Here's how the part is built. I have some questions about the finished solid (model axes, mm). Face numbers are marked on the shaded views. A direction names the side the tool comes from. Round coordinates to 2 decimals unless told otherwise and drop trailing zeros. Loops run counter-clockwise (first coordinate to the right, second up) from the corner with the lowest first, then second, coordinate; pieces in that order, holes last. Notation, with made-up numbers: M 24,72 L 58,72 A12 ccw 58,82 Z; hole C -13,-15.5 d11. An arc over 180 degrees is marked long. Write item = value, one per line. Start each with the question number.
from build123d import *

# Parameters (mm, degrees)
F0_W        = 60
F0_H        = 70
F0_W_2      = 50
F0_H_2      = 60
F1_DEPTH    = 25
F1_FACE_W   = 60
F1_FACE_H   = 70
F1_FACE_W_2 = 50
F1_FACE_H_2 = 60
F2_DEPTH    = 60
F3_R        = 5
F4_R        = 3.5
F5_DEPTH    = 70


with BuildPart() as f1:
    # F0 (on Top) → F1 (new body)
    with BuildSketch(Plane.XY):
        Rectangle(F0_W, F0_H)
        Rectangle(F0_W_2, F0_H_2, mode=Mode.SUBTRACT)
    extrude(amount=F1_DEPTH)

    # F1_face (on face) → F2 (join)
    with BuildSketch(Plane.XY.offset(25)):
        Rectangle(F1_FACE_W, F1_FACE_H)
        Rectangle(F1_FACE_W_2, F1_FACE_H_2, mode=Mode.SUBTRACT)
    extrude(amount=F2_DEPTH)

    # F3
    f3_edges = [f1.edges().sort_by_distance(p)[0] for p in [
        (25, 30, 42.5),
        (30, -35, 42.5),
        (-30, -35, 42.5),
        (-30, 35, 42.5),
        (30, 35, 42.5),
        (25, -30, 42.5),
        (-25, 30, 42.5),
        (-25, -30, 42.5),
    ]]
    fillet(f3_edges, radius=F3_R)

    # F4 (on face) → F5 (cut)
    with BuildSketch(Plane(origin=(0, 35, 0), x_dir=(-1, 0, 0), z_dir=(0, 1, 0))):
        with Locations((0, 10)):
            Circle(F4_R)
    extrude(amount=-F5_DEPTH, mode=Mode.SUBTRACT)


solid = f1.part
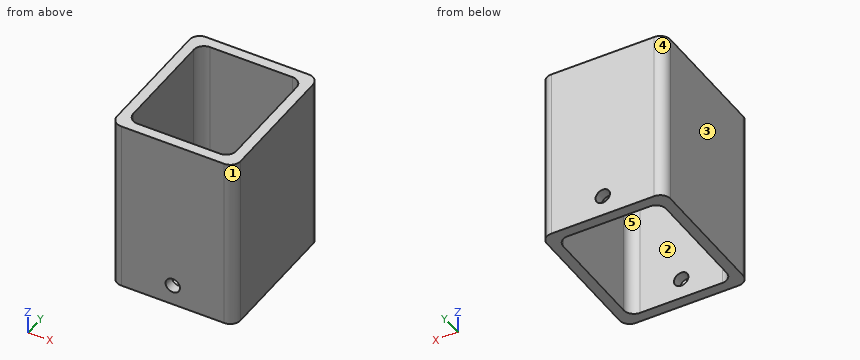
Item 1: I want a section at C-C, the plane y = 0.5. List the corners of the cut face in (x, z) for me.
Item 2: I want a section at A-A, the plane x = -6.5. List the corners of the cut face in (y, z) for me.
Item 3: For the marked faces 4 and 5, which set-ups out of +Z, -Z, +X, -X, +Y, -Y let a thin tool reach every point of the face, with its end or its side?
Item 4: I want a section at D-D, the plane x = 0. List the corners of the cut face in (y, z) for me.
Item 5: I want a section at B-B, the plane z = 10. List the corners of the cut face in (x, y) for me, then the cut area to 3 significant figures.
Item 6: Please list where these lines run through material, in increasing order: line 1 (Z direction, x = 0, y = 32); line 2 (X direction, y = -15.5, z = 59); line 3 (Y direction, x = 12, z = 63.5). Write a range as [from, to].
Item 7: We'd pull the mould along Y, two halves only. Please class the marked faces 1, 2 and 3: released by +Y, released by -Y, zero draft, split by the parting line, or undercut.
Worked out:
q1.outline = M -30,0 L -25,0 L -25,85 L -30,85 Z; M 25,0 L 30,0 L 30,85 L 25,85 Z
q2.outline = M -35,0 L -30,0 L -30,85 L -35,85 Z; M 30,0 L 35,0 L 35,85 L 30,85 Z
q3.face_4 = +Z, -Z, -X, +Y
q3.face_5 = +Z, -Z
q4.outline = M -35,0 L -30,0 L -30,6.5 L -35,6.5 Z; M -35,13.5 L -30,13.5 L -30,85 L -35,85 Z; M 30,0 L 35,0 L 35,6.5 L 30,6.5 Z; M 30,13.5 L 35,13.5 L 35,85 L 30,85 Z
q5.outline = M -30,-30 A5 ccw -25,-35 L -3.5,-35 L -3.5,-30 L -20,-30 A5 cw -25,-25 L -25,25 A5 cw -20,30 L -3.5,30 L -3.5,35 L -25,35 A5 ccw -30,30 Z; M 3.5,-35 L 25,-35 A5 ccw 30,-30 L 30,30 A5 ccw 25,35 L 3.5,35 L 3.5,30 L 20,30 A5 cw 25,25 L 25,-25 A5 cw 20,-30 L 3.5,-30 Z
q5.area = 1,130 mm2
q6.line_1 = [0, 6.5], [13.5, 85]
q6.line_2 = [-30, -25], [25, 30]
q6.line_3 = [-35, -30], [30, 35]
q7.face_1 = released by -Y
q7.face_2 = undercut
q7.face_3 = zero draft
